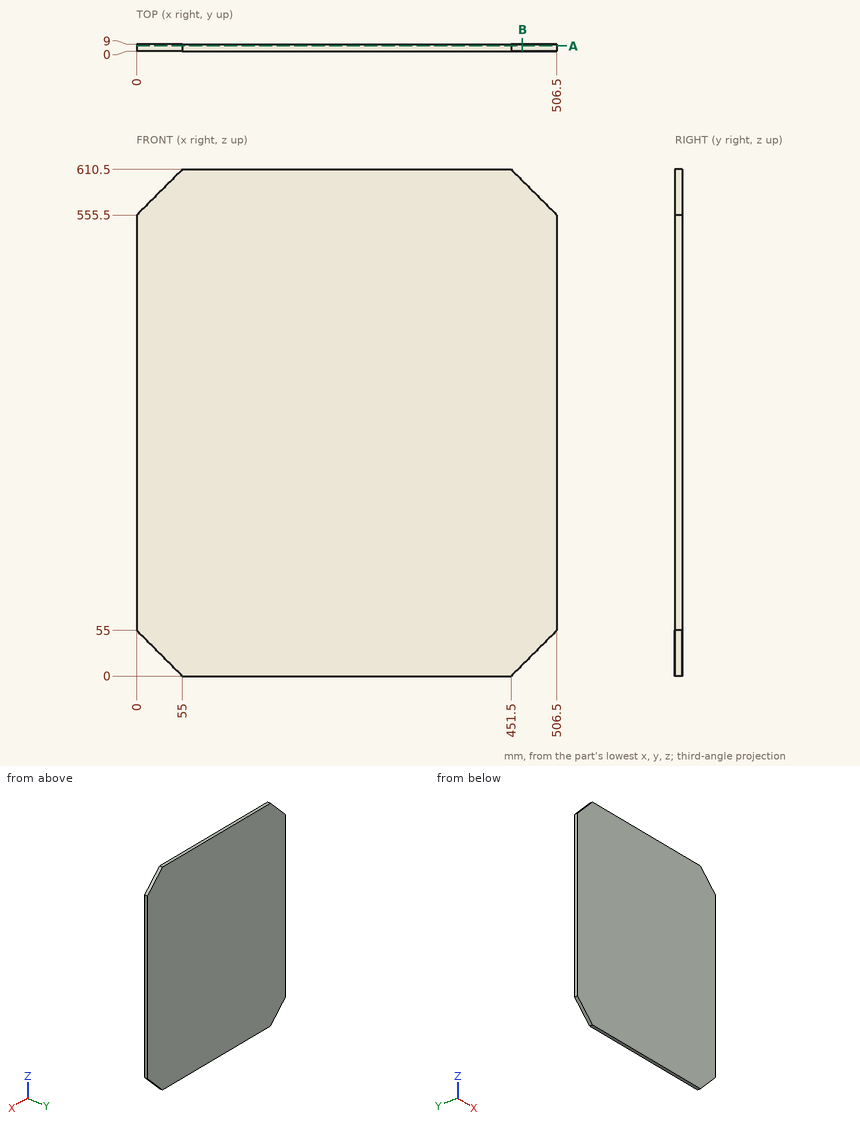
The drawing under review shows one solid part. Ordinate dimensions are in mm from its lowest x, y, z. Round coordinates to 2 decimals unless told otherwise and drop trailing zeros. Write each loop counter-clockwise with the first axis right and the second up, starting at its lowest first coordinate (ties: lowest second). Pieces come first, ordered by that corner, then holes. Notation, with made-up numbers: (61, 34) - (113, 34) arc R34 cw to (113, 68) - close; hole circle Ø8 at (-5, -12). An arc over 180 degrees is marked (long way). Use a Markdown table: item, result. Add a question column.
1. We need section A-A (y = 6.75). State the section outline as (x, z) points.
2. Wall thickness on probe 1 along X at (y, z) = (5.5, 564); probe 2 along Z at (x, y) = (467, 5.5); probe 3 along Z at (x, y) = (463.5, 0.5): over which ranges is each line inside the solid? List them lowest first.
3. We need section B-B (x = 465). State the section outline as (y, z) points.
Output:
| question | item | result |
|---|---|---|
| 1 | outline | (0, 55) - (55, 0) - (451.5, 0) - (506.5, 55) - (506.5, 555.5) - (451.5, 610.5) - (55, 610.5) - (0, 555.5) - close |
| 2 | probe 1 | x = 8.5 to 498 |
| 2 | probe 2 | z = 15.5 to 595 |
| 2 | probe 3 | z = 12 to 598.5 |
| 3 | outline | (0, 13.5) - (9, 13.5) - (9, 597) - (0, 597) - close |
